Geometry check sheet. Reference: the model listing, model coordinates, mm. Face numbers are marked on the shaded views. A direction names the side the tool comes from. Round coordinates to 2 decimals unless told otherwise and drop trailing zeros.
(1) Material ranges on line 1 along Y through (x, z) = (23.5, -15.5); line 2 along X through (y, z) = (44, -18.5); line 3 along X through (y, z) = (44, -1.75), recorded low to high.
(2) Sectioned sample at A-A (z = -3). Give the number of separate pieces and of enclosed holes in the cut face, plus the area to 3 significant figures.
(3) Go/stop test with flat-tipped pins: pin 1 (10 mm diameter, centred on x = 36, y = 61, fed in from +Z); pin 2 (12 mm diameter, centred on x = 46, y = 59.5, fed in from +Z); pin 3 (1.5 mm diameter, centred on x = 38, y = 32, fed in from +Z). Record where each tip stops, or that it passes through.
(4) Release check for a two-part mould opening along X. For the marked faces 3, 4, 5 and 6 record: +X half, -X half, draft (parallel to the pull), parting line (faces both ways), or undercut.
(5) Set-up check for the marked faces 1 and 2: record each of +Z, -Z, +X, -X, +Y, -Y from which the full face is reachable in a straight line by a thin tool's end or side.
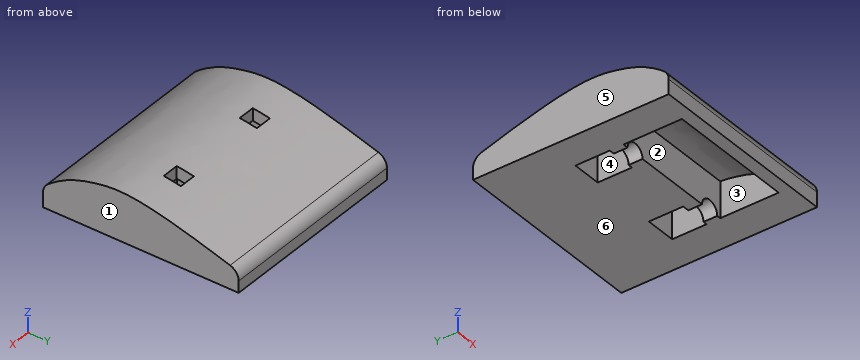
from build123d import *

# Parameters (mm, degrees)
SKETCH_1_W          = 20
SKETCH_1_H          = 80
EXTRUDE_1_DEPTH     = 80
CUT_EXTRUDE_1_DEPTH = 80
FILLET_1_R          = 5
SHELL_START         = 5
SHELL_3_DEPTH       = 70
SKETCH_3_W          = 7
SKETCH_3_H          = 7
CUT_EXTRUDE_3_DEPTH = 80
EXTRUDE_2_REACH     = 116.851
SKETCH_5_W          = 27.599035465
SKETCH_5_H          = 14.025739335
CUT_EXTRUDE_4_REACH = 99.033


# Read off the part's stored shape, not the designer's step: 쉘3
with BuildPart() as part:
    # 스케치1 → 보스-돌출1 (new body)
    with BuildSketch(Plane(origin=(0, 0, 0), x_dir=(0, 0, -1), z_dir=(1, 0, 0))):
        with Locations((10, 40)):
            Rectangle(SKETCH_1_W, SKETCH_1_H)
    extrude(amount=EXTRUDE_1_DEPTH)

    # 스케치2 → 컷-돌출1 (cut)
    with BuildSketch(Plane(origin=(80, 0, 0), x_dir=(0, 0, -1), z_dir=(1, 0, 0))):
        with BuildLine():
            Line((11.591590564, 80), (0, 80))
            Line((0, 80), (0, 0))
            Line((0, 0), (11.716359911, 0))
            add(Edge.make_bspline(
                [(11.591590564, 80), (-0.788687354, 41.111711297), (-0.930526633, 26.247395441), (4.911818792, 7.512157383), (11.716359911, 0)],
                knots=[0, 0, 0, 0, 0.618156119, 1, 1, 1, 1], degree=3))
        make_face()
    extrude(amount=-CUT_EXTRUDE_1_DEPTH, mode=Mode.SUBTRACT)

    # 필렛1
    fillet_1_edges = [part.edges().sort_by_distance(p)[0] for p in [
        (40, 0, -11.716359911),
        (40, 80, -11.591590564),
    ]]
    fillet(fillet_1_edges, radius=FILLET_1_R)

    # 쉘3 outline → 쉘3 (cut)
    with BuildSketch(Plane.YZ.offset(SHELL_START)):
        with BuildLine():
            Line((75, -20), (74.999999784, -15.255073686))
            add(Edge.make_bspline(
                [(74.999999784, -15.255073686), (67.829779133, -13.006113736), (61.460626662, -11.089637393), (55.828308111, -9.484643566), (50.869216464, -8.170232316), (46.521341581, -7.124664573), (42.721071813, -6.328318286), (39.413038096, -5.75562944), (36.528279577, -5.38717997), (34.019435823, -5.193621195), (31.801971368, -5.138118071), (29.778808064, -5.199766787), (27.603301228, -5.385408593), (27.354777332, -5.408490332), (27.107693601, -5.433274029), (26.861838696, -5.459730531), (26.617002242, -5.487832823), (26.37297533, -5.51755571), (26.129551021, -5.548875499), (25.886524852, -5.58176968), (25.643695341, -5.616216611), (25.400864489, -5.652195196), (25.157838288, -5.689684571), (24.792721691, -5.74815339), (24.670919935, -5.768015368), (24.548998185, -5.788247154), (24.426932957, -5.808846127), (24.304701052, -5.829809608), (24.182279559, -5.851134857), (24.059645852, -5.872819075), (23.936777592, -5.894859408), (23.813652725, -5.917252938), (23.690249485, -5.939996692), (23.566546391, -5.963087636), (23.380510176, -5.9982402), (23.318417709, -6.010043782), (23.256242285, -6.021932999), (23.19398134, -6.033907425), (23.131632313, -6.045966636), (23.069192642, -6.058110205), (23.006659764, -6.070337707), (22.944031116, -6.082648717), (22.881304137, -6.095042809), (22.818476264, -6.107519557), (22.755544936, -6.120078536), (22.660988915, -6.139039713), (22.629443763, -6.145380547), (22.597871828, -6.151741763), (22.566272805, -6.158123302), (22.534646389, -6.164525103), (22.502992275, -6.170947108), (22.47131016, -6.177389256), (22.439599737, -6.183851489), (22.407860702, -6.190333746), (22.376092751, -6.196835968), (22.344295578, -6.203358095), (22.28064218, -6.216442041), (22.248806222, -6.222999664), (22.216787665, -6.229608787), (22.185173002, -6.236146877), (22.153078028, -6.242800703), (22.121376446, -6.249383567), (22.089482075, -6.256023898), (22.057634411, -6.262666185), (22.025810888, -6.269319179), (21.993971685, -6.275989337), (21.962144136, -6.282671775), (21.421131548, -6.396511112), (20.913058418, -6.507182675), (20.406011367, -6.621904848), (19.899891415, -6.741190042), (19.394589314, -6.865543681), (18.889985152, -6.995466763), (18.385947953, -7.131458412), (17.882335283, -7.274018442), (17.378992852, -7.423649906), (16.875754115, -7.580861664), (16.372439878, -7.746170929), (14.987735061, -8.224441618), (14.105794888, -8.555181627), (13.222026102, -8.915168442), (12.335314555, -9.307325609), (11.444469206, -9.734725562), (10.548267461, -10.200624762), (9.645511658, -10.708471458), (8.735088494, -11.261891437), (7.816023195, -11.864657175), (6.887520219, -12.520645756), (5.94898228, -13.233790964), (4.999999509, -14.008034922)],
                knots=[0.019005596, 0.019005596, 0.019005596, 0.019005596, 0.019005596, 0.019005596, 0.019005596, 0.019005596, 0.019005596, 0.019005596, 0.019005596, 0.019005596, 0.019005596, 0.5, 0.5, 0.5, 0.5, 0.5, 0.5, 0.5, 0.5, 0.5, 0.5, 0.5, 0.5625, 0.5625, 0.5625, 0.5625, 0.5625, 0.5625, 0.5625, 0.5625, 0.5625, 0.5625, 0.5625, 0.59375, 0.59375, 0.59375, 0.59375, 0.59375, 0.59375, 0.59375, 0.59375, 0.59375, 0.59375, 0.59375, 0.609375, 0.609375, 0.609375, 0.609375, 0.609375, 0.609375, 0.609375, 0.609375, 0.609375, 0.609375, 0.609375, 0.6171875, 0.6171875, 0.6171875, 0.6171875, 0.6171875, 0.6171875, 0.6171875, 0.6171875, 0.6171875, 0.6171875, 0.6171875, 0.625, 0.625, 0.625, 0.625, 0.625, 0.625, 0.625, 0.625, 0.625, 0.625, 0.625, 0.75, 0.75, 0.75, 0.75, 0.75, 0.75, 0.75, 0.75, 0.75, 0.75, 0.75, 0.968713852, 0.968713852, 0.968713852, 0.968713852, 0.968713852, 0.968713852, 0.968713852, 0.968713852, 0.968713852, 0.968713852, 0.968713852, 0.968713852, 0.968713852], degree=12))
            Line((4.999999509, -14.008034922), (5, -20))
            Line((5, -20), (75, -20))
        make_face()
    extrude(amount=SHELL_3_DEPTH, mode=Mode.SUBTRACT)

    # 스케치3 → 컷-돌출3 (cut)
    with BuildSketch(Plane.XY):
        with Locations((19.5, 40.741655041)):
            Rectangle(SKETCH_3_W, SKETCH_3_H)
        with Locations((60.5, 40.741655041)):
            Rectangle(SKETCH_3_W, SKETCH_3_H)
    extrude(amount=-CUT_EXTRUDE_3_DEPTH, mode=Mode.SUBTRACT)

    # 스케치5 → 보스-돌출2 (add, up to next)
    with BuildSketch(Plane(origin=(0, 0, -20), x_dir=(-1, 0, 0), z_dir=(0, 0, -1)), mode=Mode.PRIVATE) as extrude_2_sk1:
        Polygon((-5, 75), (-75, 75), (-75, 48.539865482), (-65.902373449, 48.539865482), (-53.347074528, 48.539865482), (-25.748039063, 48.539865482), (-13.758294148, 48.539865482), (-5, 48.539865482), align=None)
    extrude_2_tool1 = extrude(extrude_2_sk1.sketch, amount=-EXTRUDE_2_REACH, mode=Mode.PRIVATE) - part.part
    # 스케치5 → 보스-돌출2 (add, up to next)
    with BuildSketch(Plane(origin=(0, 0, -20), x_dir=(-1, 0, 0), z_dir=(0, 0, -1)), mode=Mode.PRIVATE) as extrude_2_sk2:
        Polygon((-65.902373449, 48.539865482), (-75, 48.539865482), (-75, 5), (-65.902373449, 5), (-65.902373449, 28.858586093), (-65.902373449, 34.514126147), align=None)
    extrude_2_tool2 = extrude(extrude_2_sk2.sketch, amount=-EXTRUDE_2_REACH, mode=Mode.PRIVATE) - part.part
    # 스케치5 → 보스-돌출2 (add, up to next)
    with BuildSketch(Plane(origin=(0, 0, -20), x_dir=(-1, 0, 0), z_dir=(0, 0, -1)), mode=Mode.PRIVATE) as extrude_2_sk3:
        with Locations((-39.547556796, 41.526995814)):
            Rectangle(SKETCH_5_W, SKETCH_5_H)
    extrude_2_tool3 = extrude(extrude_2_sk3.sketch, amount=-EXTRUDE_2_REACH, mode=Mode.PRIVATE) - part.part
    # 스케치5 → 보스-돌출2 (add, up to next)
    with BuildSketch(Plane(origin=(0, 0, -20), x_dir=(-1, 0, 0), z_dir=(0, 0, -1)), mode=Mode.PRIVATE) as extrude_2_sk4:
        Polygon((-53.347074528, 34.514126147), (-65.902373449, 34.514126147), (-65.902373449, 28.858586093), (-13.758294148, 28.858586093), (-13.758294148, 34.514126147), (-25.748039063, 34.514126147), align=None)
    extrude_2_tool4 = extrude(extrude_2_sk4.sketch, amount=-EXTRUDE_2_REACH, mode=Mode.PRIVATE) - part.part
    # 스케치5 → 보스-돌출2 (add, up to next)
    with BuildSketch(Plane(origin=(0, 0, -20), x_dir=(-1, 0, 0), z_dir=(0, 0, -1)), mode=Mode.PRIVATE) as extrude_2_sk5:
        Polygon((-5, 5), (-5, 48.539865482), (-13.758294148, 48.539865482), (-13.758294148, 34.514126147), (-13.758294148, 28.858586093), (-13.758294148, 5), align=None)
    extrude_2_tool5 = extrude(extrude_2_sk5.sketch, amount=-EXTRUDE_2_REACH, mode=Mode.PRIVATE) - part.part
    add(extrude_2_tool1.solids().sort_by_distance((40, 61.769933, -20))[0])
    add(extrude_2_tool2.solids().sort_by_distance((70.451187, 26.769933, -20))[0])
    add(extrude_2_tool3.solids().sort_by_distance((39.547557, 41.526996, -20))[0])
    add(extrude_2_tool4.solids().sort_by_distance((39.830334, 31.686356, -20))[0])
    add(extrude_2_tool5.solids().sort_by_distance((9.379147, 26.769933, -20))[0])

    # 스케치6 → 컷-돌출4 (cut, up to next)
    with BuildSketch(Plane.XZ.offset(-28.858586093), mode=Mode.PRIVATE) as cut_extrude_4_sk1:
        with BuildLine():
            Line((15.927376618, -20), (23.972864062, -20))
            ThreePointArc((23.972864062, -20), (19.95012034, -15.977256278), (15.927376618, -20))
        make_face()
    cut_extrude_4_tool1 = extrude(cut_extrude_4_sk1.sketch, amount=-CUT_EXTRUDE_4_REACH, mode=Mode.PRIVATE) & part.part
    # 스케치6 → 컷-돌출4 (cut, up to next)
    with BuildSketch(Plane.XZ.offset(-28.858586093), mode=Mode.PRIVATE) as cut_extrude_4_sk2:
        with BuildLine():
            Line((56.070366463, -20), (64.284748666, -20))
            ThreePointArc((64.284748666, -20), (60.177557564, -15.892808898), (56.070366463, -20))
        make_face()
    cut_extrude_4_tool2 = extrude(cut_extrude_4_sk2.sketch, amount=-CUT_EXTRUDE_4_REACH, mode=Mode.PRIVATE) & part.part
    add(cut_extrude_4_tool1.solids().sort_by_distance((19.95012, 28.858586, -18.292695))[0], mode=Mode.SUBTRACT)
    add(cut_extrude_4_tool2.solids().sort_by_distance((60.177558, 28.858586, -18.256854))[0], mode=Mode.SUBTRACT)


solid = part.part
Answer below:
1. line 1: y = 0 to 5, 28.86 to 34.51, 48.54 to 80
1. line 2: x = 0 to 13.76, 25.75 to 53.35, 65.9 to 80
1. line 3: x = 0 to 16, 23 to 57, 64 to 80
2. separate pieces: 1
2. enclosed holes: 2
2. area: 2,730 mm2
3. pin 1: stops at z = -4.48
3. pin 2: stops at z = -3.83
3. pin 3: stops at z = -0.23
4. face 3: undercut
4. face 4: undercut
4. face 5: -X half
4. face 6: draft
5. face 1: +Z, -Z, +X, +Y, -Y
5. face 2: -Z
